Build history of the part. All positions in model axes, mm. Face numbers are marked on the shaded views. A direction names the side the tool comes from. Round coordinates to 2 decimals unless told otherwise and drop trailing zeros. Write each loop counter-clockwise with the first axis right and the second up, starting at its lowest first coordinate (ties: lowest second). Pieces come first, ordered by that corner, then holes. Notation, with made-up numbers: (-12.75, 56) -> (31.25, 56) arc R19 ccw to (31.25, 60) -> close; hole circle Ø10 at (15, 29). An arc over 180 degrees is marked (long way). One line per question, with ' | ' between items.
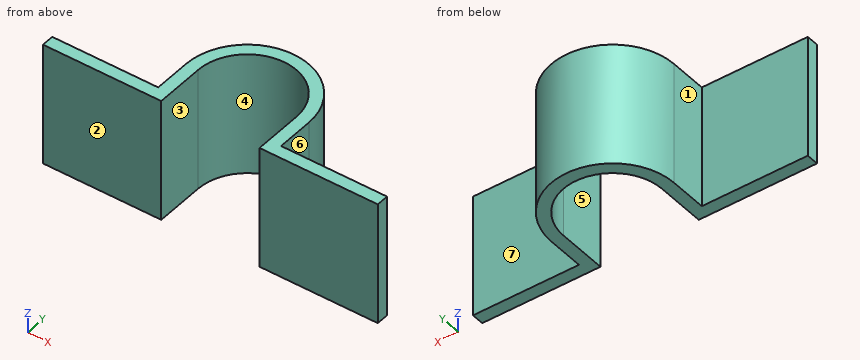
from build123d import *

# Parameters (mm, degrees)
EXTRUDE_1_DEPTH = 10


with BuildPart() as part:
    # 草图1 → 凸台-拉伸1 (new body)
    with BuildSketch(Plane.XY):
        with BuildLine():
            Line((5, 4), (5, 1))
            Line((5, 1), (13.623322376, 1))
            Line((13.623322376, 1), (13.623322376, 0))
            Line((13.623322376, 0), (4, 0))
            Line((4, 0), (4, 4))
            ThreePointArc((4, 4), (0, 8), (-4, 4))
            Line((-4, 4), (-4, 0))
            Line((-4, 0), (-13.623322376, 0))
            Line((-13.623322376, 0), (-13.623322376, 1))
            Line((-13.623322376, 1), (-5, 1))
            Line((-5, 1), (-5, 4))
            ThreePointArc((-5, 4), (0, 9), (5, 4))
        make_face()
    extrude(amount=EXTRUDE_1_DEPTH)


solid = part.part
(1) Wall check: line 1 (X direction, y = 1.5, z = 2.25); line 2 (Y direction, x = -9.25, z = 8.5); line 3 (X direction, y = 5.25, z = 5.5). Give the ranges that are in metal, low to high. Write a range as from..to.
Calculated:
line 1: -5..-4, 4..5 | line 2: 0..1 | line 3: -4.84..-3.8, 3.8..4.84
(2) Slice it at C-C (x = 2). Write the cut outline in (y, z).
Calculated:
outline: (7.46, 0) -> (8.58, 0) -> (8.58, 10) -> (7.46, 10) -> close
(3) 3-axis set-ups, long thin cutter, end or side, ignore diameter. For the marked faces 1, 2 and 3: which of +Z, -Z, +X, -X, +Y, -Y reach the whole face in a straight line?
Calculated:
face 1: +Z, -Z, -X, +Y | face 2: +Z, -Z, +X, -X, -Y | face 3: +Z, -Z, -Y
(4) Mould opens along X. For the marked faces 4, 5, 6 and 7 say: pulls with the +X half, pulls with the -X half, needs draft (parallel to the pull), parting line crosses it, or undercut.
Calculated:
face 4: undercut | face 5: undercut | face 6: pulls with the +X half | face 7: needs draft
(5) Slice it at B-B (z = 7.5). Write the cut outline in (x, y), then the cut area to 3 significant figures.
Calculated:
outline: (-13.62, 0) -> (-4, 0) -> (-4, 4) arc R4 cw to (4, 4) -> (4, 0) -> (13.62, 0) -> (13.62, 1) -> (5, 1) -> (5, 4) arc R5 ccw to (-5, 4) -> (-5, 1) -> (-13.62, 1) -> close | area: 39.4 mm2
(6) Slice it at D-D (x = -2.25). Write the cut outline in (y, z), then the cut area to 3 significant figures.
Calculated:
outline: (7.31, 0) -> (8.47, 0) -> (8.47, 10) -> (7.31, 10) -> close | area: 11.6 mm2
(7) Drop flat-ended pins along their axis: pin 1 (2.5 mm diameter, centred on x = 8.5, z = 7, fed in from +Y); pin 2 (0.9 mm diameter, centred on y = 2, z = 6, fed in from +X); pin 3 (1.5 mm diameter, centred on x = -2.5, z = 4.5, fed in from +Y). Give the stop position or say it passes through.
Calculated:
pin 1: y = 1 | pin 2: x = 5 | pin 3: y = 8.68
(8) Slice it at A-A (y = 2.75). Write the cut outline in (x, z).
Calculated:
outline: (-5, 0) -> (-4, 0) -> (-4, 10) -> (-5, 10) -> close; (4, 0) -> (5, 0) -> (5, 10) -> (4, 10) -> close
